Read the model definition and answer for the solid it produces. Units are mm, in the model's axes. A direction names the side the tool comes from. Coordinates: 2 decimals unless noted, no trailing zeros. Write each loop counter-clockwise with the first axis right and the second up, starting at its lowest first coordinate (ties: lowest second). Pieces come first, ordered by that corner, then holes.
(1) Which of the six approach directions +Z, -Z, +X, -X, +Y, -Y give full straight-line access (tool end or side, diameter ignored) to faces 1 (the flat face through (2, -9, 33.3)), 2 (the flat face through (4, -6, 45)), 3 (the cylindrical face through (-1.73, -7.81, 2.46))?
(2) The mould has two halves that part along X. Classify faces 4 (the cylindrical face through (-1.73, -7.81, 47.54)), 5 (the flat face through (4, -6, 5)), 6 (the flat face through (2, -9, 3.3)), 7 (the cylindrical face through (-8.63, 2.72, 2.64)): +X half, -X half, draft (parallel to the pull), parting line (faces both ways), or undercut.
(3) Section C-C on z = 34 is taken. Write down the section's boundary in (x, y).
(4) Find the intervals of material crossed by probe 1 along Y at (x, z) = (0, 1.95); probe 2 along Z at (x, y) = (-7, 6); probe 3 along Y at (x, z) = (0, 27), in increasing order.
(5) Given pin 1 (6 mm diameter, centred on x = -2, y = 4, fed in from +Z); pin 2 (4 mm diameter, centred on y = -5, z = 37, fed in from -X); pin 3 (6 mm diameter, centred on x = -2.5, y = 1, fed in from -Z); pin 4 (1.5 mm diameter, centred on y = -6, z = 32.5, fed in from +X), each flat-ended and moving along its own axis, determine where each tip first touches the part or whether it passes through.
(6) Section D-D on z = 40 is taken. Write down the section's boundary in (x, y), then the cut area to 3 significant figures.
from build123d import *

# Parameters (mm, degrees)
SKETCH1_R          = 10
SKETCH1_R_2        = 7
MAIN_DEPTH         = 50
SKETCH2_R          = 8
BEARING_CUT_DEPTH  = 5
SKETCH5_R          = 10
SKETCH5_R_2        = 9.05
CUT_EXTRUDE2_DEPTH = 1.3
SKETCH6_R          = 10
SKETCH6_R_2        = 9.05
CUT_EXTRUDE3_DEPTH = 1.3


with BuildPart() as part:
    # Sketch1 → Main (new body)
    with BuildSketch(Plane.XY):
        Circle(SKETCH1_R)
        Circle(SKETCH1_R_2, mode=Mode.SUBTRACT)
    extrude(amount=MAIN_DEPTH)

    # Sketch2 → Bearing Cut (cut)
    with BuildSketch(Plane.XY.offset(50)):
        Circle(SKETCH2_R)
    bearing_cut = extrude(amount=-BEARING_CUT_DEPTH, mode=Mode.SUBTRACT)

    # Mirror1: Bearing Cut across plane
    add(bearing_cut.mirror(Plane.XY.offset(25)), mode=Mode.SUBTRACT)

    # Sketch5 → Cut-Extrude2 (cut)
    with BuildSketch(Plane(origin=(0, 0, 2), x_dir=(-1, 0, 0), z_dir=(0, 0, -1))):
        Circle(SKETCH5_R)
        Circle(SKETCH5_R_2, mode=Mode.SUBTRACT)
    extrude(amount=-CUT_EXTRUDE2_DEPTH, mode=Mode.SUBTRACT)

    # Sketch6 → Cut-Extrude3 (cut)
    with BuildSketch(Plane(origin=(0, 0, 33.3), x_dir=(-1, 0, 0), z_dir=(0, 0, -1))):
        Circle(SKETCH6_R)
        Circle(SKETCH6_R_2, mode=Mode.SUBTRACT)
    extrude(amount=-CUT_EXTRUDE3_DEPTH, mode=Mode.SUBTRACT)


solid = part.part
Response:
1. face 1: none
1. face 2: +Z
1. face 3: -Z
2. face 4: undercut
2. face 5: undercut
2. face 6: draft
2. face 7: parting line
3. outline: circle Ø18.1 at (0, 0); hole circle Ø14 at (0, 0)
4. probe 1: y = -10 to -8, 8 to 10
4. probe 2: z = 0 to 2, 3.3 to 33.3, 34.6 to 50
4. probe 3: y = -10 to -7, 7 to 10
5. pin 1: stops at z = 45
5. pin 2: stops at x = -9.54
5. pin 3: passes through
5. pin 4: stops at x = 8.51
6. outline: circle Ø20 at (0, 0); hole circle Ø14 at (0, 0)
6. area: 160 mm2
